from build123d import *

# Parameters (mm, degrees)
ESQUISSE1_W        = 25
ESQUISSE1_H        = 25
ESQUISSE1_R        = 1.25
BOSS_EXTRU_2_DEPTH = 25
ESQUISSE1_5_W      = 25
ESQUISSE1_5_H      = 25
ESQUISSE1_5_R      = 1.25
BOSS_EXTRU_3_DEPTH = 25
ESQUISSE1_7_W      = 280
ESQUISSE1_7_H      = 25
BOSS_EXTRU_4_DEPTH = 10


with BuildPart() as part:
    # Esquisse1 → Boss.-Extru.2 (new body)
    with BuildSketch(Plane.XY):
        with Locations((63.75, -12.5)):
            Rectangle(ESQUISSE1_W, ESQUISSE1_H)
        with Locations((63.75, -12.5)):
            Circle(ESQUISSE1_R, mode=Mode.SUBTRACT)
    extrude(amount=BOSS_EXTRU_2_DEPTH)



with BuildPart() as body_2:
    # Esquisse1_5 → Boss.-Extru.3 (new body)
    with BuildSketch(Plane.XY):
        with Locations((216.25, -12.5)):
            Rectangle(ESQUISSE1_5_W, ESQUISSE1_5_H)
        with Locations((216.25, -12.5)):
            Circle(ESQUISSE1_5_R, mode=Mode.SUBTRACT)
    extrude(amount=BOSS_EXTRU_3_DEPTH)


with BuildPart() as part_1:
    add(part.part)

    add(body_2.part)  # Boss.-Extru.4 merges body 2
    # Esquisse1_7 → Boss.-Extru.4 (add)
    with BuildSketch(Plane.XY):
        with Locations((140, 12.5)):
            Rectangle(ESQUISSE1_7_W, ESQUISSE1_7_H)
    extrude(amount=BOSS_EXTRU_4_DEPTH)


solid = part_1.part
For this review, take the finished solid that the model builds, in its own axes (mm). A direction names the side the tool comes from. Round coordinates to 2 decimals unless told otherwise and drop trailing zeros. Order: outer loops, then holes, each group sorted by start corner. A loop starts at its lowest first (then second) coordinate and runs counter-clockwise, first axis right, second up. Notation, with made-up numbers: (-21.75, 61) -> (16.25, 61) arc R3 cw to (16.25, 66) -> close; hole circle Ø8 at (21.5, 76.25). An arc over 180 degrees is marked (long way). Put each result on its own line as item: value.
Q1. Mouldability with a two-part tool opening along X and no side actions: class faces 1 (the flat face through (203.75, -13, 12)), 2 (the flat face through (139, 0, 5)), 3 (the flat face through (61, -12, 25)), 4 (the flat face through (280, 12, 5)) as pulls with the +X half, pulls with the -X half, needs draft (parallel to the pull), parting line crosses it, or undercut.
Check result:
face 1: undercut
face 2: undercut
face 3: needs draft
face 4: pulls with the +X half
Q2. Add section C-C on x = 241.5. Write out the cut boundary in (y, z).
Check result:
outline: (0, 0) -> (25, 0) -> (25, 10) -> (0, 10) -> close
Q3. For probe 1 along X at (y, z) = (-21.5, 2.25); probe 2 along Y at (x, z) = (216.25, 13.5); probe 3 along Y at (x, z) = (216.25, 8.5), list the stretches that pass through material, from the lowest coordinate up. Write a range as [from, to].
Check result:
probe 1: [51.25, 76.25], [203.75, 228.75]
probe 2: [-25, -13.75], [-11.25, 0]
probe 3: [-25, -13.75], [-11.25, 25]
Q4. Machinability: for faces 5 (the flat face through (76.25, -13, 12)), 6 (the flat face through (64, 0, 17)), 7 (the flat face through (254, 0, 5)), which of the approach directions +Z, -Z, +X, -X, +Y, -Y give a long, thin tool a straight path to every point of the face, cutting with its end or side? Answer none if there is none.
Check result:
face 5: +Z, -Z, -Y
face 6: +Z, +X, -X, +Y
face 7: +Z, -Z, +X, -Y
Q5. Add section A-A on z = 12.5. Write out the cut boundary in (x, y), plus the area to 3 significant figures.
Check result:
outline: (51.25, -25) -> (76.25, -25) -> (76.25, 0) -> (51.25, 0) -> close; (203.75, -25) -> (228.75, -25) -> (228.75, 0) -> (203.75, 0) -> close; hole circle Ø2.5 at (63.75, -12.5); hole circle Ø2.5 at (216.25, -12.5)
area: 1,240 mm2
Q6. Insertion check: pin 1 Ø1 at (x, y) = (85.5, 4.5) entering from +Z; pin 2 Ø8 at (x, z) = (137.5, 3) entering from -Y; pin 3 Ø4.5 at (x, z) = (215.5, 15.5) entering from +Y. Each pin has a flat end and moves straight along its axis. Give the tip position at first contact, or say it passes through.
Check result:
pin 1: z = 10
pin 2: y = 0
pin 3: y = 0
Q7. Add section B-B on y = -18. Write out the cut boundary in (x, z).
Check result:
outline: (51.25, 0) -> (76.25, 0) -> (76.25, 25) -> (51.25, 25) -> close; (203.75, 0) -> (228.75, 0) -> (228.75, 25) -> (203.75, 25) -> close
